from build123d import *

# Parameters (mm, degrees)
F0_R     = 6.35
F1_DEPTH = 12.7
F2_DEPTH = 114.3
F4_DEPTH = 73.0029466568
F3_R     = 12.7
F5_DEPTH = 73.0029466568
F6_DEPTH = 114.301


with BuildPart() as f1:
    # F0 (on Top) → F1 (new body)
    with BuildSketch(Plane.XY):
        Polygon((0, 88.9), (0, 0), (31.75, 0), (63.5, 0), (63.5, 88.9), align=None)
        with Locations((12.7, 11.43)):
            Circle(F0_R, mode=Mode.SUBTRACT)
        with Locations((50.8, 11.43)):
            Circle(F0_R, mode=Mode.SUBTRACT)
        Polygon((57.9139342054, 43.5440988757), (31.75, 0), (20.8639752811, 6.5409835514), (47.0279094865, 50.085082427), align=None, mode=Mode.SUBTRACT)
        with Locations((12.7, 77.47)):
            Circle(F0_R, mode=Mode.SUBTRACT)
        with Locations((50.8, 77.47)):
            Circle(F0_R, mode=Mode.SUBTRACT)
        with Locations((50.8, 77.47)):
            Circle(F0_R)
        with Locations((12.7, 77.47)):
            Circle(F0_R)
        Polygon((20.8639752811, 6.5409835514), (31.75, 0), (57.9139342054, 43.5440988757), (47.0279094865, 50.085082427), align=None)
        with Locations((50.8, 11.43)):
            Circle(F0_R)
        with Locations((12.7, 11.43)):
            Circle(F0_R)
    extrude(amount=F1_DEPTH)

    # F0 (on Top) → F2 (join)
    with BuildSketch(Plane.XY):
        Polygon((20.8639752811, 6.5409835514), (31.75, 0), (57.9139342054, 43.5440988757), (47.0279094865, 50.085082427), align=None)
    extrude(amount=F2_DEPTH)

    # F3 (on face) → F4 (cut, through all)
    with BuildSketch(Plane(origin=(23.3278610592, -14.0167930366, 0), x_dir=(0.5150380749, 0.8571673007, 0), z_dir=(0.8571673007, -0.5150380749, 0))):
        with BuildLine():
            Line((16.3524588784, 114.3), (16.3524588784, 88.9))
            ThreePointArc((16.3524588784, 88.9), (23.7919466363, 106.8605122421), (41.7524588784, 114.3))
            Line((41.7524588784, 114.3), (16.3524588784, 114.3))
        make_face()
        with BuildLine():
            Line((67.1524588784, 114.3), (41.7524588784, 114.3))
            ThreePointArc((41.7524588784, 114.3), (59.7129711205, 106.8605122421), (67.1524588784, 88.9))
            Line((67.1524588784, 88.9), (67.1524588784, 114.3))
        make_face()
    extrude(amount=-F4_DEPTH, mode=Mode.SUBTRACT)

    # F3 (on face) → F5 (cut, through all)
    with BuildSketch(Plane(origin=(23.3278610592, -14.0167930366, 0), x_dir=(0.5150380749, 0.8571673007, 0), z_dir=(0.8571673007, -0.5150380749, 0))):
        with Locations((41.7524588784, 88.9)):
            Circle(F3_R)
    extrude(amount=-F5_DEPTH, mode=Mode.SUBTRACT)

    # F0 (on Top) → F6 (cut, through all)
    with BuildSketch(Plane.XY):
        with Locations((50.8, 11.43)):
            Circle(F0_R)
        with Locations((50.8, 77.47)):
            Circle(F0_R)
        with Locations((12.7, 77.47)):
            Circle(F0_R)
        with Locations((12.7, 11.43)):
            Circle(F0_R)
    extrude(amount=F6_DEPTH, mode=Mode.SUBTRACT)


solid = f1.part
Design review of the part built by this model. Coordinates are the model's own, in mm. A direction names the side the tool comes from. Give positions to 0.01 mm unless a question says otherwise; leave off trailing zeros. Write each loop counter-clockwise with the first axis right and the second up, starting at its lowest first coordinate (ties: lowest second). Pieces come first, ordered by that corner, then holes. Notation, with made-up numbers: M 48.5,36 L 104.5,36 A27 ccw 104.5,56 Z; hole C 61.5,74.5 d8. An arc over 180 degrees is marked long. Answer as a JSON object with one key per item and string values. Group by question number.
1) We need section B-B (x = 12.7). Give the boundary of the cut face in (y, z), and give its area (3 significant figures).
2) For line 1 along X through (y, z) = (11.43, 8.25); line 2 along Y through (x, z) = (12.7, 5); line 3 along Y through (x, z) = (12, 10), list the stretches that pass through material, from the lowest coordinate up.
3) We need section D-D (y = 67). Give the boundary of the cut face in (x, z), and give its area (3 significant figures).
4) Clearance check with flat-ended pins moving along their axes: pin 1 Ø5 at (x, y) = (35, 40) entering from +Z; pin 2 Ø1 at (y, z) = (46, 44.5) entering from +X; pin 3 Ø2 at (y, z) = (32, 84) entering from +X. State where each tip first meets the part, or that it passes through.
5) Tool access review of faces 5 (the face through (26.231, 3.316, 50.267)), 6 (the face through (34.13, 28.62, 62.79)), 7 (the face through (31, 0, 6)), 8 (the face through (52.547, 46.769, 50.267)): name each direction out of +Z, -Z, +X, -X, +Y, -Y from which nothing blocks a thin tool from reaching the whole face with its end or side.
6) We need section A-A (y = 77.47). Give the boundary of the cut face in (x, z).
7) Mouldability with a two-part tool opening along Y and no side actions: class faces 1 (the face through (44.65, 21.47, 62.79)), 2 (the face through (31, 45, 0)), 3 (the face through (38.61, 23.58, 101.49)), 4 (the face through (54.214, 82.824, 6.261)) as released by +Y, released by -Y, zero draft, split by the parting line, or undercut.
8) We need section C-C (z = 95). Give the boundary of the cut face in (x, y).
Answer key:
{
 "1": {"outline": "M 0,0 L 5.08,0 L 5.08,12.7 L 0,12.7 Z; M 17.78,0 L 71.12,0 L 71.12,12.7 L 17.78,12.7 Z; M 83.82,0 L 88.9,0 L 88.9,12.7 L 83.82,12.7 Z", "area": "806 mm²"},
 "2": {"line 1": "x = 0 to 6.35, 19.05 to 44.45, 57.15 to 63.5", "line 2": "y = 0 to 5.08, 17.78 to 71.12, 83.82 to 88.9", "line 3": "y = 0 to 5.12, 17.74 to 71.16, 83.78 to 88.9"},
 "3": {"outline": "M 0,0 L 63.5,0 L 63.5,12.7 L 0,12.7 Z", "area": "806 mm²"},
 "4": {"pin 1": "stops at z = 12.7", "pin 2": "stops at x = 54.66", "pin 3": "stops at x = 51.58"},
 "5": {"face 5": "+Z, -X, -Y", "face 6": "+Z, -X, +Y", "face 7": "+Z, -Z, +X, -X, -Y", "face 8": "+Z, +X, +Y"},
 "6": {"outline": "M 0,0 L 6.35,0 L 6.35,12.7 L 0,12.7 Z; M 19.05,0 L 44.45,0 L 44.45,12.7 L 19.05,12.7 Z; M 57.15,0 L 63.5,0 L 63.5,12.7 L 57.15,12.7 Z"},
 "7": {"face 1": "released by -Y", "face 2": "zero draft", "face 3": "undercut", "face 4": "undercut"},
 "8": {"outline": "M 21.25,7.18 L 32.13,0.64 L 39.09,12.22 L 28.21,18.76 Z; M 39.68,37.86 L 50.57,31.32 L 57.53,42.91 L 46.65,49.45 Z"}
}
